Autodesk Inventor part; units mm, degrees
ref_plane "YZ Plane" through (0, 0, 0) normal (1, 0, 0) x (0, 1, 0)
ref_plane "XZ Plane" through (0, 0, 0) normal (0, 1, 0) x (-1, 0, 0)
ref_plane "XY Plane" through (0, 0, 0) normal (0, 0, 1) x (1, 0, 0)
sketch "Sketch1" plane through (0, 0, 0) normal (0, 0, 1) x (1, 0, 0)
  arc A0 (49.1564, -72.9751) -> (-49.1564, -72.9751) centre (0, -254.0664) ccw
  line L0 (49.1564, -72.9751) -> (73.0086, -49.1229)
  line L1 (86.9345, 13.6367) -> (74.7113, 47.4192)
  line L2 (74.7113, 47.4192) -> (49.163, 72.9816)
  line L3 (-49.163, 72.9816) -> (-75.1179, 47.041)
  line L4 (-75.1179, 47.041) -> (-86.9513, 13.6826)
  line L5 (-49.1564, -72.9751) -> (-73.0086, -49.1229)
  arc A1 (-49.163, 72.9816) -> (49.163, 72.9816) centre (0, 254.0664) ccw
  arc A2 (-73.0086, -49.1229) -> (-86.9513, 13.6826) centre (-146.4572, -32.478) ccw
  arc A3 (86.9345, 13.6367) -> (73.0086, -49.1229) centre (146.4645, -32.4974) ccw
  line L6 (0, 0) -> (0, -66.422)
  line L7 (0, 0) -> (0, 66.4266)
  line L8 (78.5091, -0.0284) -> (-78.4957, -0.0284)
  line L9 (-49.163, 72.9816) -> (49.163, 72.9816)
  line L10 (-49.163, 72.9816) -> (-31.7513, 72.9816)
  line L11 (-31.7513, 72.9816) -> (-31.7513, -69.1278)
  line L12 (49.163, 72.9816) -> (31.7513, 72.9816)
  line L13 (31.7513, 72.9816) -> (31.7513, -69.1278)
  line L14 (31.7513, -69.1278) -> (31.7513, 95.9722)
  line L15 (31.7513, 95.9722) -> (-31.7513, 95.9722)
  line L16 (-31.7513, 95.9722) -> (-31.7513, 72.9816)
  line L17 (31.7513, -69.1278) -> (31.7513, -81.8278)
  line L18 (31.7513, -81.8278) -> (-31.7513, -81.8278)
  line L19 (-31.7513, -81.8278) -> (-31.7513, -69.1278)
  line L20 (31.7513, 95.9722) -> (34.9263, 95.9722)
  line L21 (34.9263, 95.9722) -> (34.9263, -81.8278)
  line L22 (34.9263, -81.8278) -> (31.7513, -81.8278)
  line L23 (-31.7513, 95.9722) -> (-34.9263, 95.9722)
  line L24 (-34.9263, 95.9722) -> (-34.9263, -81.8278)
  line L25 (-34.9263, -81.8278) -> (-31.7513, -81.8278)
  line L26 (31.7513, 95.9722) -> (31.7513, 92.7972)
  line L27 (31.7513, 92.7972) -> (-31.7513, 92.7972)
extrude "Extrusion1" add sketch "Sketch1" along normal blind 3.175 contours L17 L18 L19 A0 | L13 L8 L21 A0 | A0 L6 L8 L13 | A0 L21 L22 L17 | A0 L11 L8 L6 | L13 A1 L21 L8 | L8 L6 L7 A1 L13 | L19 L25 L24 A0 | A0 L24 L8 L11 | L8 L11 A1 L7 L6 | L13 L9 L21 A1 | A1 L11 L9 L13 | L8 L24 A1 L11 | L14 L20 L21 L9 | L9 L16 L27 L14 | A1 L24 L9 L11 | L9 L24 L23 L16 | L27 L16 L15 L14
sketch "Sketch2" plane through (0, 0, 3.175) normal (0, 0, 1) x (1, 0, 0)
  line L0 (34.9263, 95.9722) -> (-34.9263, 95.9722)
  line L1 (-34.9263, 95.9722) -> (-34.9263, -81.8278)
  line L2 (-34.9263, -81.8278) -> (34.9263, -81.8278)
  line L3 (34.9263, -81.8278) -> (34.9263, 95.9722)
  line L4 (-34.9263, 95.9722) -> (-34.9263, 92.7972)
  line L5 (-34.9263, 92.7972) -> (34.9263, 92.7972)
  line L6 (34.9263, -81.8278) -> (31.7513, -81.8278)
  line L7 (31.7513, -81.8278) -> (31.7513, 92.7972)
  line L8 (-34.9263, -81.8278) -> (-31.7513, -81.8278)
  line L9 (-31.7513, -81.8278) -> (-31.7513, 92.7972)
  point P0 (0, 0)
  dimension "d9" = 3.175
  dimension "d10" = 3.175
  dimension "d11" = 3.175
extrude "Extrusion2" add sketch "Sketch2" along normal blind 28.575 contours L3 L5 L1 L0 | L3 L2 L7 L5 | L5 L9 L2 L1
sketch "Sketch3" plane through (-31.7513, 92.7972, 3.175) normal (0, -1, 0) x (1, 0, 0)
  line L0 (63.5025, 0) -> (63.5025, 28.575)
  line L1 (0, 28.575) -> (63.5025, 28.575)
  line L2 (0, 28.575) -> (0, 0)
  line L3 (63.5025, 28.575) -> (63.5025, 25.4)
  line L4 (63.5025, 25.4) -> (0, 25.4)
  point P0 (31.7513, -3.175)
  dimension "d14" = 3.175
extrude "Extrusion3" add sketch "Sketch3" along normal blind 28.575
sketch "Sketch4" plane through (34.9263, -81.8278, 0) normal (1, 0, 0) x (0, 0, -1)
  line L0 (-31.75, 0) -> (-31.75, 177.8)
  line L1 (0, 0) -> (-31.75, 0)
  line L2 (-31.75, 0) -> (-31.75, 135.5494)
  line L3 (-31.75, 135.5494) -> (-10.3194, 135.5494)
  line L4 (-10.3194, 135.5494) -> (-10.3194, 0)
  point P0 (0, 81.8278)
extrude "Extrusion4" cut sketch "Sketch4" against normal blind 127
sketch "Sketch5" plane through (34.9263, -81.8278, 10.3194) normal (0, 0, 1) x (1, 0, 0)
  line L0 (-3.175, 0) -> (-3.175, 135.5494)
  line L1 (0, 0) -> (-3.175, 0)
  line L2 (0, 135.5494) -> (0, 0)
  line L3 (0, 0) -> (0, 25.4)
  line L4 (0, 25.4) -> (-3.175, 25.4)
  point P0 (-34.9263, 81.8278)
  dimension "d19" = 25.4
sketch "Sketch6" plane through (-34.9263, 53.7216, 10.3194) normal (0, 0, 1) x (1, 0, 0)
  line L0 (3.175, 0) -> (3.175, -135.5494)
  line L1 (0, -135.5494) -> (0, 0)
  line L2 (3.175, -135.5494) -> (0, -135.5494)
  line L3 (3.175, -135.5494) -> (3.175, -110.1494)
  line L4 (3.175, -110.1494) -> (0, -110.1494)
  point P0 (34.9263, -53.7216)
  dimension "d20" = 25.4
extrude "Extrusion5" add sketch "Sketch6" along normal blind 28.575
extrude "Extrusion6" add sketch "Sketch5" along normal blind 28.575
sketch "Sketch7" plane through (31.7513, -81.8278, 3.175) normal (-1, 0, 0) x (0, 0, 1)
  line L0 (0, 0) -> (35.7194, 0)
  line L1 (35.7194, 25.4) -> (35.7194, 0)
  line L2 (7.1444, 25.4) -> (35.7194, 25.4)
  line L3 (35.7194, 25.4) -> (32.5444, 25.4)
  line L4 (32.5444, 25.4) -> (32.5444, 0)
  point P0 (-3.175, 81.8278)
  dimension "d25" = 3.175
extrude "Extrusion7" add sketch "Sketch7" along normal blind 66.04
chamfer "Chamfer1" distance 2.54 angle 45 5 edges at (0, 95.9722, 31.75) (-34.9263, 95.9722, 15.875) (0, 92.7972, 3.175) (34.9263, 95.9722, 15.875) (0, 95.9722, 0)
chamfer "Chamfer2" distance 2.54 angle 45 4 edges at (0, -81.8278, 38.8944) (0, -81.8278, 0) (-34.9263, -81.8278, 19.4472) (34.9263, -81.8278, 19.4472)
properties part number "Battery Holder"
Here's how the part is built. I have some questions about the finished solid (model axes, mm). A direction names the side the tool comes from. Round coordinates to 2 decimals unless told otherwise and drop trailing zeros. Write each loop counter-clockwise with the first axis right and the second up, starting at its lowest first coordinate (ties: lowest second). Pieces come first, ordered by that corner, then holes. Notation, with made-up numbers: (42.25, 23.5) -> (101.25, 23.5) arc R29 ccw to (101.25, 47.5) -> close; hole circle Ø10 at (-30.5, -9). An arc over 180 degrees is marked (long way). One line per item, written item: value.
1) We'd pull the mould along X, two halves only. Please class faces 6 (the face through (-34.926, 6, 6)), 7 (the face through (0, -68, 38.894)), 8 (the face through (0, 92.797, 17)): released by +X, released by -X, zero draft, split by the parting line, or undercut.
Filled sheet:
face 6: released by -X
face 7: zero draft
face 8: undercut
2) Suppose I cut it at B-B on z = 23.5. List the corners of the cut face in (x, y) for me, plus the area to 3 significant figures.
Filled sheet:
outline: (-34.93, -79.29) -> (-32.39, -81.83) -> (-31.75, -81.83) -> (-31.75, -56.43) -> (-34.93, -56.43) -> close; (-34.93, 53.72) -> (-31.75, 53.72) -> (-31.75, 92.8) -> (31.75, 92.8) -> (31.75, 53.72) -> (34.93, 53.72) -> (34.93, 93.43) -> (32.39, 95.97) -> (-32.39, 95.97) -> (-34.93, 93.43) -> close; (31.75, -81.83) -> (32.39, -81.83) -> (34.93, -79.29) -> (34.93, -56.43) -> (31.75, -56.43) -> close
area: 618 mm2
3) For faces 1 (the face through (0, 95.972, 16)), 2 (the face through (0, 64.222, 30)), 3 (the face through (0, -69, 35.719)), 4 (the face through (0, 79, 28.575)), 5 (the face through (33, -1, 10.319)), which set-ups out of +Z, -Z, +X, -X, +Y, -Y let a thin tool reach every point of the face, with its end or its side?
Filled sheet:
face 1: +Z, -Z, +X, -X, +Y
face 2: +Z, -Y
face 3: +Y, -Y
face 4: -Y
face 5: +Z, +X, -X
4) If I drill on line 1 (Z direction, x = -6.5, y = 89.5) (3 decimals); line 2 (X direction, y = 79.5, z = 20); line 3 (Z direction, x = -30.5, y = 15.5) (3 decimals), over which ranges is the centre line in solid material (lowest first)? Write a range as [from, to].
Filled sheet:
line 1: z = [0, 3.175], [28.575, 31.75]
line 2: x = [-34.93, -31.75], [31.75, 34.93]
line 3: z = [0, 3.175]
5) Suppose I cut it at D-D on y = -6. List the corners of the cut face in (x, z) for me (3 decimals), plus the area to 3 significant figures.
Filled sheet:
outline: (-34.926, 0) -> (34.926, 0) -> (34.926, 10.319) -> (31.751, 10.319) -> (31.751, 3.175) -> (-31.751, 3.175) -> (-31.751, 10.319) -> (-34.926, 10.319) -> close
area: 267 mm2
6) Suppose I cut it at A-A on x = 13. List the corners of the cut face in (y, z) for me (3 decimals).
Filled sheet:
outline: (-81.828, 2.54) -> (-79.288, 0) -> (93.432, 0) -> (95.972, 2.54) -> (95.972, 29.21) -> (93.432, 31.75) -> (64.222, 31.75) -> (64.222, 28.575) -> (92.797, 28.575) -> (92.797, 5.715) -> (90.257, 3.175) -> (-81.828, 3.175) -> close; (-81.828, 35.719) -> (-56.428, 35.719) -> (-56.428, 38.894) -> (-79.288, 38.894) -> (-81.828, 36.354) -> close
7) Suppose I cut it at C-C on y = -62. List the corners of the cut face in (x, z) for me (3 decimals).
Filled sheet:
outline: (-34.926, 0) -> (34.926, 0) -> (34.926, 38.894) -> (-34.926, 38.894) -> close; hole (-31.751, 3.175) -> (31.751, 3.175) -> (31.751, 35.719) -> (-31.751, 35.719) -> close
8) I'm going to push flat-ended pins straight in: pin 1 Ø1.5 at (x, y) = (-11.5, -27.5) entering from +Z (3 decimals); pin 2 Ø1 at (x, z) = (10.5, 31) entering from -Y; pin 3 Ø4 at (x, z) = (19, 7) entering from -Y; pin 4 Ø16.5 at (y, z) = (5.5, 21) entering from +X. Where does each tip first touch, or does it pass through?
Filled sheet:
pin 1: stops at z = 3.175
pin 2: stops at y = 64.22
pin 3: stops at y = 92.08
pin 4: passes through
